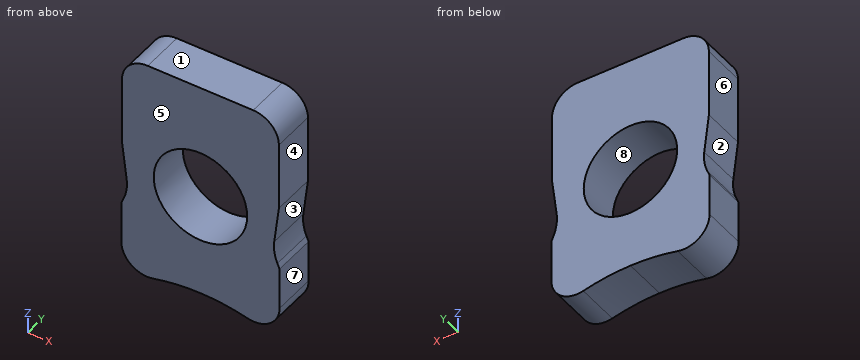
```python
from build123d import *

# Parameters (mm, degrees)
F0_R     = 21.45
F1_DEPTH = 20


with BuildPart() as f1:
    # F0 (on Front) → F1 (new body)
    with BuildSketch(Plane.XZ):
        with BuildLine():
            Line((24.2, 53.5), (-24.2, 53.5))
            ThreePointArc((-24.2, 53.5), (-32.54386, 50.04386), (-36, 41.7))
            Line((-36, 41.7), (-36, 10.541781))
            Line((-36, 10.541781), (-33.86535, -6.843548))
            ThreePointArc((-33.86535, -6.843548), (-33.914779, -11.969259), (-35.298202, -16.904995))
            Line((-35.298202, -16.904995), (-36.299529, -19.24014))
            Line((-36.299529, -19.24014), (-36.299529, -38.57162))
            ThreePointArc((-36.299529, -38.57162), (-31.817885, -47.933904), (-21.673998, -50.133694))
            ThreePointArc((-21.673998, -50.133694), (-10.916713, -48.160836), (0, -47.5))
            ThreePointArc((0, -47.5), (10.916713, -48.160836), (21.673998, -50.133694))
            ThreePointArc((21.673998, -50.133694), (31.817885, -47.933904), (36.299529, -38.57162))
            Line((36.299529, -38.57162), (36.299529, -19.24014))
            Line((36.299529, -19.24014), (35.298202, -16.904995))
            ThreePointArc((35.298202, -16.904995), (33.914779, -11.969259), (33.86535, -6.843548))
            Line((33.86535, -6.843548), (36, 10.541781))
            Line((36, 10.541781), (36, 41.7))
            ThreePointArc((36, 41.7), (32.54386, 50.04386), (24.2, 53.5))
        make_face()
        Circle(F0_R, mode=Mode.SUBTRACT)
    extrude(amount=F1_DEPTH)


solid = f1.part
```
Check sheet for the modelled part. Datum: model origin and axes. Units: mm. Face numbers are marked on the shaded views. A direction names the side the tool comes from. Round coordinates to 2 decimals unless told otherwise and drop trailing zeros. Write each loop counter-clockwise with the first axis right and the second up, starting at its lowest first coordinate (ties: lowest second). Pieces come first, ordered by that corner, then holes. Notation, with made-up numbers: (-36.5, -24) -> (12.5, -24) arc R23 cw to (12.5, 11) -> close; hole circle Ø2 at (85.5, 7). An arc over 180 degrees is marked (long way). One line per question, with ' | ' between items. Start each with the question number.
1. Scan lines: line 1 along Z through (x, y) = (-4.5, -15.5); line 2 along Z through (x, y) = (-9, -6); line 3 along X through (y, z) = (-11, -1). Record each from-to range of solid material in increasing order. Write a range as from..to.
2. Sectioned sample at D-D, the plane x = 30.5. Record the cut outline in (y, z), then the cut area to 3 significant figures.
3. Set-up check for the marked faces 1, 2, 3 and 4: record each of +Z, -Z, +X, -X, +Y, -Y from which the full face is reachable in a straight line by a thin tool's end or side.
4. Sectioned sample at B-B, the plane z = -9.5. Record the cut outline in (x, y).
5. Release check for a two-part mould opening along X. For the marked faces 5, 6, 7 and 8 record: +X half, -X half, draft (parallel to the pull), parting line (faces both ways), or undercut.
6. Depth check by flat-ended pin: pin 1 (1 mm diameter, centred on x = 3, y = -11, fed in from -Z); pin 2 (3 mm diameter, centred on x = -14.5, y = -4.5, fed in from -Z); pin 3 (1.5 mm diameter, centred on y = -15, z = 33.5, fed in from +X). Enter the tip coordinate at first touch or a pass-through.
7. Sectioned sample at A-A, the plane x = -9. Record the cut outline in (y, z), then the cut area to 3 significant figures.
8. Sectioned sample at C-C, the plane y = -10.5. Record the cut outline in (x, z) (3 decimals), then the cut area to 3 significant figures.
Taken from the geometry:
1) line 1: z = -47.61..-20.97, 20.97..53.5 | line 2: z = -47.95..-19.47, 19.47..53.5 | line 3: x = -34.58..-21.43, 21.43..34.58
2) outline: (-20, -48.84) -> (0, -48.84) -> (0, 51.68) -> (-20, 51.68) -> close | area: 2,010 mm^2
3) face 1: +Z, +X, -X, +Y, -Y | face 2: -X, +Y, -Y | face 3: +X, +Y, -Y | face 4: +Z, +X, +Y, -Y
4) outline: (-33.72, -20) -> (-19.23, -20) -> (-19.23, 0) -> (-33.72, 0) -> close; (19.23, -20) -> (33.72, -20) -> (33.72, 0) -> (19.23, 0) -> close
5) face 5: draft | face 6: -X half | face 7: +X half | face 8: undercut
6) pin 1: stops at z = -47.57 | pin 2: stops at z = -48.93 | pin 3: stops at x = 36
7) outline: (-20, -47.95) -> (0, -47.95) -> (0, -19.47) -> (-20, -19.47) -> close; (-20, 19.47) -> (0, 19.47) -> (0, 53.5) -> (-20, 53.5) -> close | area: 1,250 mm^2
8) outline: (-36.3, -38.572) arc R11.8 ccw to (-21.674, -50.134) arc R90.5 cw to (0, -47.5) arc R90.5 cw to (21.674, -50.134) arc R11.8 ccw to (36.3, -38.572) -> (36.3, -19.24) -> (35.298, -16.905) arc R19.5 cw to (33.865, -6.844) -> (36, 10.542) -> (36, 41.7) arc R11.8 ccw to (24.2, 53.5) -> (-24.2, 53.5) arc R11.8 ccw to (-36, 41.7) -> (-36, 10.542) -> (-33.865, -6.844) arc R19.5 cw to (-35.298, -16.905) -> (-36.3, -19.24) -> close; hole circle Ø42.9 at (0, 0) | area: 5,770 mm^2
